Could you check a few things on this model? Use its own coordinates, in mm. A direction names the side the tool comes from. Round coordinates to 2 decimals unless told otherwise and drop trailing zeros. Order: outer loops, then holes, each group sorted by start corner. A loop starts at its lowest first (then second) coordinate and runs counter-clockwise, first axis right, second up.
```python
from build123d import *

# Parameters (mm, degrees)
SKETCH_W        = 60
SKETCH_H        = 75
PAD_DEPTH       = 10
POCKET_DEPTH    = 4
SKETCH002_R     = 3.003779
SKETCH002_W     = 16.509998
SKETCH002_H     = 13.460002
POCKET001_DEPTH = 5


with BuildPart() as part:
    # Sketch → Pad (new body)
    with BuildSketch(Plane.XY):
        Rectangle(SKETCH_W, SKETCH_H)
    extrude(amount=PAD_DEPTH)

    # Sketch001 (on Face6 of Pad) → Pocket (cut)
    with BuildSketch(Plane.XY.offset(10)):
        with BuildLine():
            Line((-26.160018, 34.131806), (25.909982, 34.131806))
            ThreePointArc((28.449982, 31.591806), (27.706037, 33.38786), (25.909982, 34.131806))
            Line((28.449982, 31.591806), (28.449982, -13.493194))
            ThreePointArc((25.274982, -16.668194), (27.520043, -15.738255), (28.449982, -13.493194))
            Line((-26.160018, -16.668194), (25.274982, -16.668194))
            ThreePointArc((-28.700018, -14.128194), (-27.956072, -15.924248), (-26.160018, -16.668194))
            Line((-28.700018, 31.591806), (-28.700018, -14.128194))
            ThreePointArc((-26.160018, 34.131806), (-27.956078, 33.387866), (-28.700018, 31.591806))
        make_face()
    extrude(amount=-POCKET_DEPTH, mode=Mode.SUBTRACT)

    # Sketch002 (on Face3 of Pocket) → Pocket001 (cut)
    with BuildSketch(Plane.YZ.offset(30)):
        with Locations((3.362204, 11.229303)):
            Circle(SKETCH002_R)
        with Locations((-9.887796, 11.229303)):
            Circle(SKETCH002_R)
        with Locations((18.913807, 14.92554)):
            Rectangle(SKETCH002_W, SKETCH002_H)
    extrude(amount=-POCKET001_DEPTH, mode=Mode.SUBTRACT)


solid = part.part
```
Q1. We'd pull the mould along X, two halves only. Please class faces 1 (the flat face through (29, 8, 10)), 2 (the flat face through (-30, -1, 5)), 3 (the flat face through (0, 9, 6)): released by +X, released by -X, zero draft, split by the parting line, or undercut.
Q2. Imagine slicing it at B-B, the plane z = 7.25. Please give me the cut outline in (x, y).
Q3. For faces 4 (the flat face through (0, 37.5, 5)), 5 (the flat face through (28.45, 9, 8)), 6 (the cylindrical face through (29.236, -9.936, 8.226)), which set-ups out of +Z, -Z, +X, -X, +Y, -Y let a thin tool reach every point of the face, with its end or its side?
Q4. I need wall thicknesses on L1, parallel to Y at x = 22.5, z = 6.5; L2, parallel to X at y = 4, z = 6.75; L3, parallel to Z at x = 22.5, y = 27. Which ranges of each line are inside material? Lowest first, please.
Q5. For P1, Ø8, axis at x = 0.5, y = 10.5, coming from the +Z side; P2, Ø1.2, axis at x = 29.5, y = 16.5, coming from the +Z side, each with a flat end and sliding along its axis, tell me the tip position at first contact or that it passes through.
Q6. Imagine slicing it at A-A, the plane y = -2. Please give me the cut outline in (x, z).
Q7. Imagine slicing it at C-C, the plane x = 21.5. Please give me the cut outline in (y, z), then the cut area to 3 significant figures.
Filled in:
1. face 1: zero draft
1. face 2: released by -X
1. face 3: undercut
2. outline: (-30, -37.5) - (30, -37.5) - (30, 37.5) - (-30, 37.5) - close; hole (-28.7, -14.13) arc R2.54 ccw to (-26.16, -16.67) - (25.27, -16.67) arc R3.18 ccw to (28.45, -13.49) - (28.45, 31.59) arc R2.54 ccw to (25.91, 34.13) - (-26.16, 34.13) arc R2.54 ccw to (-28.7, 31.59) - close
3. face 4: +Z, -Z, +X, -X, +Y
3. face 5: +Z
3. face 6: +Z, +X
4. L1: y = -37.5 to -16.67, 34.13 to 37.5
4. L2: x = -30 to -28.7, 28.45 to 30
4. L3: z = 0 to 6
5. P1: stops at z = 6
5. P2: stops at z = 8.2
6. outline: (-30, 0) - (30, 0) - (30, 10) - (28.45, 10) - (28.45, 6) - (-28.7, 6) - (-28.7, 10) - (-30, 10) - close
7. outline: (-37.5, 0) - (37.5, 0) - (37.5, 10) - (34.13, 10) - (34.13, 6) - (-16.67, 6) - (-16.67, 10) - (-37.5, 10) - close
7. area: 547 mm2
